Part model, mm, in its own coordinate system. Face numbers are marked on the shaded views. A direction names the side the tool comes from. Coordinates: 2 decimals unless noted, no trailing zeros. Order: outer loops, then holes, each group sorted by start corner. A loop starts at its lowest first (then second) coordinate and runs counter-clockwise, first axis right, second up. Notation, with made-up numbers: (5, 45) - (25, 45) arc R28 ccw to (25, 81) - close; hole circle Ø9 at (69.5, 33.5). An arc over 180 degrees is marked (long way). Use a Markdown table: item, result. Add a question column.
1) Saw through at C-C on y = -32. List the corners of the cut face in (x, z).
2) Saw through at B-B on z = 268. List the corners of the cut face in (x, y), then the cut area to 3 significant figures.
3) Drop flat-ended pins along their axis: P1, Ø8, axis at x = 44, y = -40, coming from the +Z side; P2, Ø11, axis at x = 4, z = 297, coming from the +Y side; P3, Ø3, axis at y = -7, z = 419, coming from the +X side; P4, Ø5.5, axis at x = -44.45, y = -44.45, coming from the -Z side. Give the stop position or say it passes through.
4) Tool access for the marked faces 1, 2 and 3: list every direction of +Z, -Z, +X, -X, +Y, -Y with a clear straight run to the whole face (end or side of a thin tool).
5) Wall check: L1, parallel to X at y = -44, z = 3; L2, parallel to Y at x = 44.45, z = 3.25 (3 decimals); L3, parallel to X at y = 10, z = 488. Give the ranges that are in metal, low to high. Write a range as [from, to].
6) Saw through at A-A on y = 0. List the corners of the cut face in (x, z), then the cut area to 3 significant figures.
```python
from build123d import *

# Parameters (mm, degrees)
F0_W     = 114.3
F0_H     = 114.3
F0_R     = 3.175
F1_DEPTH = 6.35
F2_W     = 50.8
F2_H     = 50.8
F2_W_2   = 47.625
F2_H_2   = 47.625
F3_DEPTH = 533.4
F4_R     = 5.08
F6_DEPTH = 82.551


with BuildPart() as f1:
    # F0 (on Top) → F1 (new body)
    with BuildSketch(Plane.XY):
        Rectangle(F0_W, F0_H)
        with Locations((-44.45, -44.45)):
            Circle(F0_R, mode=Mode.SUBTRACT)
        with Locations((44.45, -44.45)):
            Circle(F0_R, mode=Mode.SUBTRACT)
        with Locations((-44.45, 44.45)):
            Circle(F0_R, mode=Mode.SUBTRACT)
        with Locations((44.45, 44.45)):
            Circle(F0_R, mode=Mode.SUBTRACT)
    extrude(amount=F1_DEPTH)

    # F2 (on face) → F3 (join)
    with BuildSketch(Plane.XY.offset(6.35)):
        Rectangle(F2_W, F2_H)
        Rectangle(F2_W_2, F2_H_2, mode=Mode.SUBTRACT)
    extrude(amount=F3_DEPTH)

    # F4
    f4_edges = [f1.edges().sort_by_distance(p)[0] for p in [
        (25.4, 25.4, 273.05),
        (25.4, -25.4, 273.05),
        (-25.4, 25.4, 273.05),
        (-25.4, -25.4, 273.05),
        (-23.8125, -23.8125, 273.05),
        (23.8125, 23.8125, 273.05),
        (-23.8125, 23.8125, 273.05),
        (23.8125, -23.8125, 273.05),
    ]]
    fillet(f4_edges, radius=F4_R)

    # F5 (on face) → F6 (cut, through all)
    with BuildSketch(Plane(origin=(-25.4, 0, 0), x_dir=(0, -1, 0), z_dir=(-1, 0, 0))):
        with BuildLine():
            ThreePointArc((-6.35, 50.8), (0, 44.45), (6.35, 50.8))
            Line((6.35, 50.8), (6.35, 457.2))
            ThreePointArc((6.35, 457.2), (0, 463.55), (-6.35, 457.2))
            Line((-6.35, 457.2), (-6.35, 50.8))
        make_face()
    extrude(amount=-F6_DEPTH, mode=Mode.SUBTRACT)


solid = f1.part
```
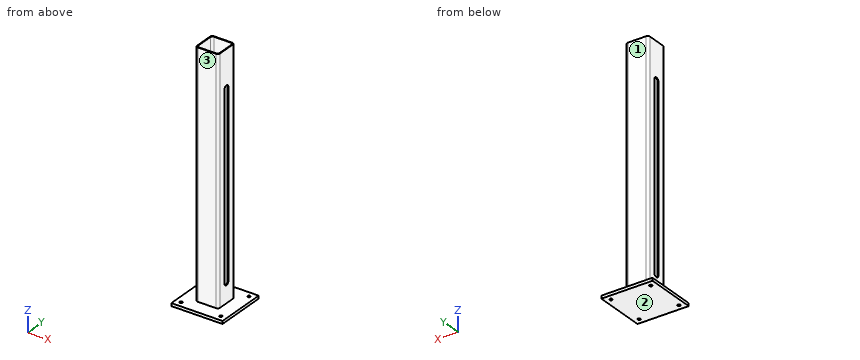
Results are:
| question | item | result |
|---|---|---|
| 1 | outline | (-57.15, 0) - (57.15, 0) - (57.15, 6.35) - (-57.15, 6.35) - close |
| 2 | outline | (-25.4, -20.32) arc R5.08 ccw to (-20.32, -25.4) - (20.32, -25.4) arc R5.08 ccw to (25.4, -20.32) - (25.4, -6.35) - (23.81, -6.35) - (23.81, -18.73) arc R5.08 cw to (18.73, -23.81) - (-18.73, -23.81) arc R5.08 cw to (-23.81, -18.73) - (-23.81, -6.35) - (-25.4, -6.35) - close; (-25.4, 6.35) - (-23.81, 6.35) - (-23.81, 18.73) arc R5.08 cw to (-18.73, 23.81) - (18.73, 23.81) arc R5.08 cw to (23.81, 18.73) - (23.81, 6.35) - (25.4, 6.35) - (25.4, 20.32) arc R5.08 ccw to (20.32, 25.4) - (-20.32, 25.4) arc R5.08 ccw to (-25.4, 20.32) - close |
| 2 | area | 272 mm2 |
| 3 | P1 | z = 6.35 |
| 3 | P2 | y = 25.4 |
| 3 | P3 | x = 25.4 |
| 3 | P4 | through |
| 4 | face 1 | +Z, +X, -X, +Y |
| 4 | face 2 | -Z, +X, -X, +Y, -Y |
| 4 | face 3 | +Z, +X, -X, -Y |
| 5 | L1 | [-57.15, -47.59], [-41.31, 41.31], [47.59, 57.15] |
| 5 | L2 | [-57.15, -47.625], [-41.275, 41.275], [47.625, 57.15] |
| 5 | L3 | [-25.4, -23.81], [23.81, 25.4] |
| 6 | outline | (-57.15, 0) - (57.15, 0) - (57.15, 6.35) - (25.4, 6.35) - (25.4, 44.45) - (23.81, 44.45) - (23.81, 6.35) - (-23.81, 6.35) - (-23.81, 44.45) - (-25.4, 44.45) - (-25.4, 6.35) - (-57.15, 6.35) - close; (-25.4, 463.55) - (-23.81, 463.55) - (-23.81, 539.75) - (-25.4, 539.75) - close; (23.81, 463.55) - (25.4, 463.55) - (25.4, 539.75) - (23.81, 539.75) - close |
| 6 | area | 1,090 mm2 |
